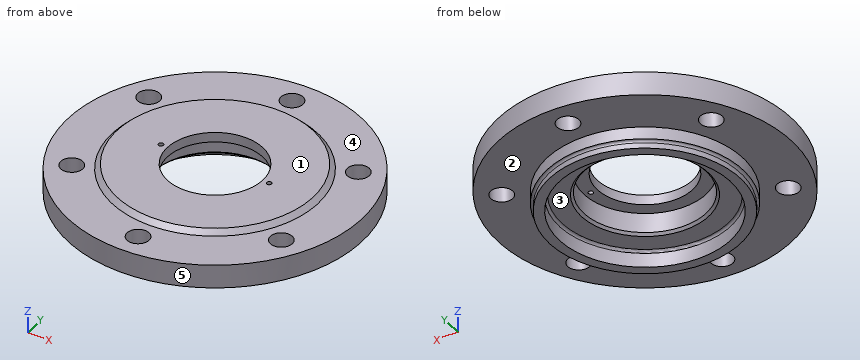
```python
from build123d import *

# Parameters (mm, degrees)
CUT_EXTRUDE1_REACH = 88.71
SKETCH6_R          = 4.5
CUT_EXTRUDE2_REACH = 89.144
SKETCH10_R         = 1


with BuildPart() as part:
    # Sketch1 → Revolve1 (revolve)
    with BuildSketch(Plane(origin=(0, 0, 0), x_dir=(0, 0, -1), z_dir=(1, 0, 0)), mode=Mode.PRIVATE) as revolve1_sk:
        with BuildLine():
            Line((0, 19.5), (0, 40))
            Line((0, 40), (2, 42))
            Line((2, 42), (2, 60))
            Line((2, 60), (11.6, 60))
            Line((11.6, 60), (11.6, 40))
            Line((11.6, 40), (16.6, 40))
            ThreePointArc((16.6, 40), (16.892893219, 39.292893219), (17.6, 39))
            Line((17.6, 39), (19.85, 39))
            Line((19.85, 39), (19.85, 35))
            Line((19.85, 35), (14, 35))
            ThreePointArc((14, 35), (13.292893219, 34.707106781), (13, 34))
            Line((13, 34), (13, 26))
            Line((13, 26), (12, 25))
            Line((12, 25), (4, 25))
            Line((4, 25), (4, 19.5))
            Line((4, 19.5), (0, 19.5))
        make_face()
    revolve(revolve1_sk.sketch.rotate(Axis((0, 0, 0), (0, 0, -1)), 90), axis=Axis((0, 0, 0), (0, 0, -1)))

    # Sketch6 → Cut-Extrude1 (cut, up to next)
    with BuildSketch(Plane.XY.offset(-2), mode=Mode.PRIVATE) as cut_extrude1_sk1:
        with Locations((0, -50)):
            Circle(SKETCH6_R)
    cut_extrude1_tool1 = extrude(cut_extrude1_sk1.sketch, amount=-CUT_EXTRUDE1_REACH, mode=Mode.PRIVATE) & part.part
    # Sketch6 → Cut-Extrude1 (cut, up to next)
    with BuildSketch(Plane.XY.offset(-2), mode=Mode.PRIVATE) as cut_extrude1_sk2:
        with Locations((-43.301270189, -25)):
            Circle(SKETCH6_R)
    cut_extrude1_tool2 = extrude(cut_extrude1_sk2.sketch, amount=-CUT_EXTRUDE1_REACH, mode=Mode.PRIVATE) & part.part
    # Sketch6 → Cut-Extrude1 (cut, up to next)
    with BuildSketch(Plane.XY.offset(-2), mode=Mode.PRIVATE) as cut_extrude1_sk3:
        with Locations((-43.301270189, 25)):
            Circle(SKETCH6_R)
    cut_extrude1_tool3 = extrude(cut_extrude1_sk3.sketch, amount=-CUT_EXTRUDE1_REACH, mode=Mode.PRIVATE) & part.part
    # Sketch6 → Cut-Extrude1 (cut, up to next)
    with BuildSketch(Plane.XY.offset(-2), mode=Mode.PRIVATE) as cut_extrude1_sk4:
        with Locations((0, 50)):
            Circle(SKETCH6_R)
    cut_extrude1_tool4 = extrude(cut_extrude1_sk4.sketch, amount=-CUT_EXTRUDE1_REACH, mode=Mode.PRIVATE) & part.part
    # Sketch6 → Cut-Extrude1 (cut, up to next)
    with BuildSketch(Plane.XY.offset(-2), mode=Mode.PRIVATE) as cut_extrude1_sk5:
        with Locations((43.301270189, 25)):
            Circle(SKETCH6_R)
    cut_extrude1_tool5 = extrude(cut_extrude1_sk5.sketch, amount=-CUT_EXTRUDE1_REACH, mode=Mode.PRIVATE) & part.part
    # Sketch6 → Cut-Extrude1 (cut, up to next)
    with BuildSketch(Plane.XY.offset(-2), mode=Mode.PRIVATE) as cut_extrude1_sk6:
        with Locations((43.301270189, -25)):
            Circle(SKETCH6_R)
    cut_extrude1_tool6 = extrude(cut_extrude1_sk6.sketch, amount=-CUT_EXTRUDE1_REACH, mode=Mode.PRIVATE) & part.part
    add(cut_extrude1_tool1.solids().sort_by_distance((0, -50, -2))[0], mode=Mode.SUBTRACT)
    add(cut_extrude1_tool2.solids().sort_by_distance((-43.30127, -25, -2))[0], mode=Mode.SUBTRACT)
    add(cut_extrude1_tool3.solids().sort_by_distance((-43.30127, 25, -2))[0], mode=Mode.SUBTRACT)
    add(cut_extrude1_tool4.solids().sort_by_distance((0, 50, -2))[0], mode=Mode.SUBTRACT)
    add(cut_extrude1_tool5.solids().sort_by_distance((43.30127, 25, -2))[0], mode=Mode.SUBTRACT)
    add(cut_extrude1_tool6.solids().sort_by_distance((43.30127, -25, -2))[0], mode=Mode.SUBTRACT)

    # Sketch10 → Cut-Extrude2 (cut, up to next)
    with BuildSketch(Plane.XY, mode=Mode.PRIVATE) as cut_extrude2_sk1:
        with Locations((-22.36, 0)):
            Circle(SKETCH10_R)
    cut_extrude2_tool1 = extrude(cut_extrude2_sk1.sketch, amount=-CUT_EXTRUDE2_REACH, mode=Mode.PRIVATE) & part.part
    # Sketch10 → Cut-Extrude2 (cut, up to next)
    with BuildSketch(Plane.XY, mode=Mode.PRIVATE) as cut_extrude2_sk2:
        with Locations((22.36, 0)):
            Circle(SKETCH10_R)
    cut_extrude2_tool2 = extrude(cut_extrude2_sk2.sketch, amount=-CUT_EXTRUDE2_REACH, mode=Mode.PRIVATE) & part.part
    add(cut_extrude2_tool1.solids().sort_by_distance((-22.36, 0, 0))[0], mode=Mode.SUBTRACT)
    add(cut_extrude2_tool2.solids().sort_by_distance((22.36, 0, 0))[0], mode=Mode.SUBTRACT)


solid = part.part
```
Part model, mm, in its own coordinate system. Face numbers are marked on the shaded views. A direction names the side the tool comes from. Give positions to 0.01 mm unless a question says otherwise; leave off trailing zeros. Write each loop counter-clockwise with the first axis right and the second up, starting at its lowest first coordinate (ties: lowest second). Pieces come first, ordered by that corner, then holes. Notation, with made-up numbers: (-16.5, -24.5) -> (40.5, -24.5) arc R10 ccw to (40.5, -12.5) -> close; hole circle Ø7 at (-5, 12.5). An arc over 180 degrees is marked (long way). Put each result on its own line as item: value. Start each with the question number.
Item 1: Cut at B-B (y = 50). List the corners of the cut face in (x, z).
Item 2: Which spindle directions (+Z, -Z, +X, -X, +Y, -Y) get a long thin tool onto all of the face, cutting with end or side? Do the marked faces 1 and 2. Say none if no direction does.
Item 3: Pin check, flat tips, straight feed: pin 1 Ø20.5 at (x, y) = (-15, -13.5) entering from -Z; pin 2 Ø5 at (x, z) = (46, -11.5) entering from +Y; pin 3 Ø6 at (y, z) = (-14.5, -4) entering from +X. Stop position of each tip, or through.
Item 4: Pull direction X, two halves, no side cores. Call the marked faces 3, 4 and 5: pulls with the +X half, pulls with the -X half, needs draft (parallel to the pull), parting line crosses it, or undercut.
Item 5: Wall check: L1, parallel to Y at x = 0, z = -6.25; L2, parallel to Y at x = 0, z = -18.55; L3, parallel to Y at x = 42, z = -5.5. Give the ranges that are in metal, low to high. Write a range as [from, to].
Item 6: Cut at A-A (x = 0). State how many separate pieces and enclosed holes the cut face has, then the cut area to 3 significant figures.
Answer list:
1. outline: (-33.17, -11.6) -> (-4.5, -11.6) -> (-4.5, -2) -> (-33.17, -2) -> close; (4.5, -11.6) -> (33.17, -11.6) -> (33.17, -2) -> (4.5, -2) -> close
2. face 1: +Z, +X, -X, +Y, -Y
2. face 2: -Z
3. pin 1: stops at z = -13
3. pin 2: stops at y = 41.32
3. pin 3: stops at x = 58.89
4. face 3: undercut
4. face 4: needs draft
4. face 5: parting line crosses it
5. L1: y = [-60, -54.5], [-45.5, -25], [25, 45.5], [54.5, 60]
5. L2: y = [-39, -35], [35, 39]
5. L3: y = [-42.85, -29.31], [-20.69, 20.69], [29.31, 42.85]
6. separate pieces: 4
6. enclosed holes: 0
6. area: 711 mm2
